Source: CAD feature listing. Evaluate the final solid. Frame: model axes, mm. Face numbers are marked on the shaded views. A direction names the side the tool comes from. Coordinates: 2 decimals unless noted, no trailing zeros. Loops run counter-clockwise (first coordinate to the right, second up) from the corner with the lowest first, then second, coordinate; pieces in that order, holes last. Notation, with made-up numbers: (80.25, 30.25) -> (90.25, 30.25) arc R35 ccw to (90.25, 65.25) -> close; hole circle Ø5 at (-35.5, 59). An arc over 180 degrees is marked (long way). One line per question, with ' | ' between items. Start each with the question number.
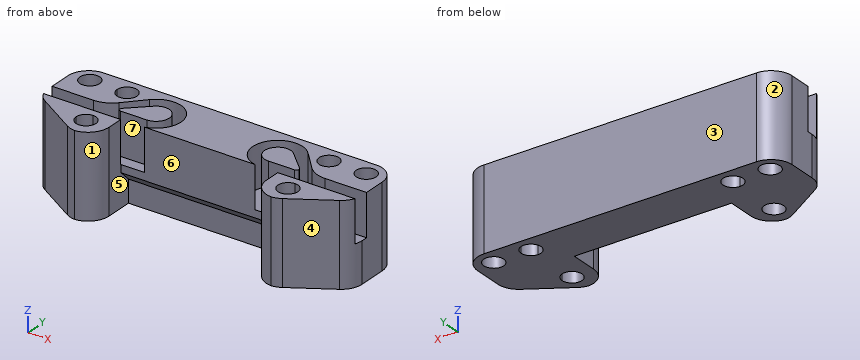
```python
from build123d import *

# Parameters (mm, degrees)
F1_DEPTH    = 15.7
F2_W        = 10.0960650777
F2_H        = 2.7
F3_DEPTH    = 8
F4_R        = 5
F5_T1_DEPTH = 26.8923143391
F5_T3_DEPTH = 21.3473434867
F5_T5_DEPTH = 35.7
F6_W        = 15
F6_H        = 6.25
F7_DEPTH    = 2
F8_SIZE     = 1.99999


# Not quite as in the source:
# - a fillet or chamfer that OpenCascade refuses, or shapes differently, is made with other operations: its cross-section is extruded or revolved along the edge and cut away or added
# - a fillet or chamfer is up to 0.001 mm smaller than in the source, because OpenCascade refuses the exact size


with BuildPart() as f1:
    # F0 (on Top) → F1 (new body)
    with BuildSketch(Plane.XY):
        Polygon((30, 9), (0, 9), (0, -1.8), (15, -1.8), (15, -9), (19.5954625243, -9), (30, -2.6151265483), align=None)
        with BuildLine():
            ThreePointArc((21.17, -5.2), (17.9264971157, -6.5435028843), (19.27, -3.3))
            ThreePointArc((19.27, -3.3), (20.6135028843, -3.8564971157), (21.17, -5.2))
        make_face(mode=Mode.SUBTRACT)
        with BuildLine():
            ThreePointArc((19.27, 3.9), (17.9264971157, 7.1435028843), (21.17, 5.8))
            ThreePointArc((21.17, 5.8), (20.6135028843, 4.4564971157), (19.27, 3.9))
        make_face(mode=Mode.SUBTRACT)
        with BuildLine():
            ThreePointArc((24.47, 5.8), (26.37, 7.7), (28.27, 5.8))
            ThreePointArc((28.27, 5.8), (26.37, 3.9), (24.47, 5.8))
        make_face(mode=Mode.SUBTRACT)
    extrude(amount=F1_DEPTH)

    # F2 (on face) → F3 (cut)
    with BuildSketch(Plane.XY.offset(15.7)):
        with BuildLine():
            ThreePointArc((11.6039349223, 0.3250306588), (9.2827431951, 3.7535073497), (13.3280728534, 4.6353754864))
            Line((13.3280728534, 4.6353754864), (16.2527744297, 1.8499454137))
            ThreePointArc((16.2527744297, 1.8499454137), (16.328577113, 2.3348713274), (16.3539349223, 2.8250306588))
            ThreePointArc((16.3539349223, 2.8250306588), (16.0328522645, 4.5417691876), (15.1130123218, 6.0264172029))
            ThreePointArc((15.1130123218, 6.0264172029), (7.5069370658, 5.2285923001), (10.5215341623, -1.8))
            Line((10.5215341623, -1.8), (12.6863356823, -1.8))
            ThreePointArc((12.6863356823, -1.8), (14.376262754, -1.0320016711), (15.6428085277, 0.3250306588))
            Line((15.6428085277, 0.3250306588), (11.6039349223, 0.3250306588))
        make_face()
        with BuildLine():
            ThreePointArc((16.3539349223, 2.8250306588), (16.328577113, 2.3348713274), (16.2527744297, 1.8499454137))
            Line((16.2527744297, 1.8499454137), (16.9487625085, 1.1870996243))
            ThreePointArc((16.9487625085, 1.1870996243), (17.0635074373, 1.0219903081), (17.1039349223, 0.8250306588))
            ThreePointArc((17.1039349223, 0.8250306588), (16.9574883129, 0.4714772682), (16.6039349223, 0.3250306588))
            Line((16.6039349223, 0.3250306588), (15.6428085277, 0.3250306588))
            ThreePointArc((15.6428085277, 0.3250306588), (14.376262754, -1.0320016711), (12.6863356823, -1.8))
            Line((12.6863356823, -1.8), (15, -1.8))
            Line((15, -1.8), (15, -1.9249693412))
            Line((15, -1.9249693412), (19.9039349223, -1.9249693412))
            Line((19.9039349223, -1.9249693412), (19.9039349223, 0.7750306588))
            Line((19.9039349223, 0.7750306588), (15.1130123218, 6.0264172029))
            ThreePointArc((15.1130123218, 6.0264172029), (16.0328522645, 4.5417691876), (16.3539349223, 2.8250306588))
        make_face()
        with Locations((24.9519674612, -0.5749693412)):
            Rectangle(F2_W, F2_H)
    extrude(amount=-F3_DEPTH, mode=Mode.SUBTRACT)

    # F4
    f4_edges = [f1.edges().sort_by_distance(p)[0] for p in [
        (19.903935, 0.775031, 11.7),
    ]]
    fillet(f4_edges, radius=F4_R)

    # F5: fillet of radius 4 on 4 edges, made by hand

    # F5_s2 → F5_t1 (cut)
    with BuildSketch(Plane.XY.offset(-5.5961571696)):
        with BuildLine():
            ThreePointArc((30, -0.3766636805), (29.4905957559, -2.3300559271), (28.0921293656, -3.7859150232))
            Line((28.0921293656, -3.7859150232), (30, -2.6151265483))
            Line((30, -2.6151265483), (30, -0.3766636805))
        make_face()
    extrude(amount=F5_T1_DEPTH, mode=Mode.SUBTRACT)

    # F5_s4 → F5_t3 (cut)
    with BuildSketch(Plane.XY.offset(-2.8236717433)):
        with BuildLine():
            ThreePointArc((20.5581231925, -8.4092513427), (19.5529608525, -8.8494808332), (18.465993827, -9))
            Line((18.465993827, -9), (19.5954625243, -9))
            Line((19.5954625243, -9), (20.5581231925, -8.4092513427))
        make_face()
    extrude(amount=F5_T3_DEPTH, mode=Mode.SUBTRACT)

    # F5_s6 → F5_t5 (cut)
    with BuildSketch(Plane.XY.offset(-10)):
        with BuildLine():
            ThreePointArc((15, -5), (16.1715728753, -7.8284271247), (19, -9))
            Line((19, -9), (15, -9))
            Line((15, -9), (15, -5))
        make_face()
        with BuildLine():
            ThreePointArc((30, 5), (28.8284271247, 7.8284271247), (26, 9))
            Line((26, 9), (30, 9))
            Line((30, 9), (30, 5))
        make_face()
    extrude(amount=F5_T5_DEPTH, mode=Mode.SUBTRACT)

    # F6 (on face) → F7 (cut)
    with BuildSketch(Plane.XZ.offset(1.8)):
        with Locations((7.5, 3.125)):
            Rectangle(F6_W, F6_H)
    extrude(amount=-F7_DEPTH, mode=Mode.SUBTRACT)

    # F8 (size 2 in the source; OpenCascade refuses exactly that, so slightly less here)
    f8_edges = [f1.edges().sort_by_distance(p)[0] for p in [
        (7.5, 0.2, 6.25),
    ]]
    chamfer(f8_edges, length=F8_SIZE)

    # F9: F1 across plane


with BuildPart() as f1_1:
    add(f1.part)
    add(f1.part.mirror(Plane.YZ))


solid = f1_1.part
```
(1) Cut plane C-C, the plane x = -20. Return the cut outline in (y, z).
(2) Draft query along X for the marked faces 1, 2 and 3. Return one class per face: pulls with the +X half, pulls with the -X half, needs draft (parallel to the pull), parting line crosses it, or undercut.
(3) Ray query, L1, parallel to X at y = 4.5, z = 5.25; L2, parallel to X at y = 6.5, z = 6.25; L3, parallel to X at y = -6.5, z = 5.75. Return the intervals inside material, ascending.
(4) Contact query for flat-ended pins moving along their axis: pin 1 Ø4 at (x, z) = (-14.5, 12.5) entering from -Y; pin 2 Ø4 at (x, z) = (4.5, 12.5) entering from -Y; pin 3 Ø3 at (x, y) = (-19.27, -5.2) entering from +Z. Output: stop coordinate, or through.
(5) Access query for the marked faces 4, 5, 6 and 7. Directions: +Z, -Z, +X, -X, +Y, -Y. A direction counts if a zero-diameter tool reaches every point of the face in a straight line with its end or side. Return the directions, or none.
(6) Cut plane A-A, the plane z = 3.25. Return the cut outline in (x, y).
Here are the results:
1) outline: (-8.69, 0) -> (-6.95, 0) -> (-6.95, 15.7) -> (-8.69, 15.7) -> close; (-3.45, 0) -> (4.05, 0) -> (4.05, 15.7) -> (1.24, 15.7) -> (1.24, 7.7) -> (-1.92, 7.7) -> (-1.92, 15.7) -> (-3.45, 15.7) -> close; (7.55, 0) -> (9, 0) -> (9, 15.7) -> (7.55, 15.7) -> close
2) face 1: undercut | face 2: pulls with the -X half | face 3: needs draft
3) L1: x = -30 to -27.76, -24.98 to -20.66, -17.88 to 17.88, 20.66 to 24.98, 27.76 to 30 | L2: x = -29.71 to -28.14, -24.6 to -21.04, -17.5 to 17.5, 21.04 to 24.6, 28.14 to 29.71 | L3: x = -23.67 to -20.66, -17.88 to -15.29, 15.29 to 17.88, 20.66 to 23.67
4) pin 1: stops at y = -8.12 | pin 2: stops at y = -1.8 | pin 3: passes through
5) face 4: +Z, -Z, +X, -Y | face 5: -Z, -Y | face 6: +Z, -Z, -Y | face 7: +Z, -X
6) outline: (-30, -0.38) arc R4 ccw to (-28.09, -3.79) -> (-20.56, -8.41) arc R4 ccw to (-18.73, -8.99) arc R4 ccw to (-15, -5) -> (-15, 0.2) -> (15, 0.2) -> (15, -5) arc R4 ccw to (18.73, -8.99) arc R4 ccw to (20.56, -8.41) -> (28.09, -3.79) arc R4 ccw to (30, -0.38) -> (30, 5) arc R4 ccw to (26, 9) -> (-26, 9) arc R4 ccw to (-30, 5) -> close; hole circle Ø3.8 at (-26.37, 5.8); hole circle Ø3.8 at (-19.27, -5.2); hole circle Ø3.8 at (-19.27, 5.8); hole circle Ø3.8 at (19.27, -5.2); hole circle Ø3.8 at (19.27, 5.8); hole circle Ø3.8 at (26.37, 5.8)
